from build123d import *

# Parameters (mm, degrees)
SKETCH1_R           = 150
SKETCH1_R_2         = 1.25
SKETCH1_R_3         = 1
SKETCH1_W           = 2
SKETCH1_H           = 4
BOSS_EXTRUDE1_DEPTH = 3.175
SKETCH2_R           = 1.4224
CUT_EXTRUDE1_DEPTH  = 10


with BuildPart() as part:
    # Sketch1 → Boss-Extrude1 (new body)
    with BuildSketch(Plane(origin=(0, 0, 0), x_dir=(1, 0, 0), z_dir=(0, 1, 0))):
        with Locations((106.066017178, 106.066017178)):
            Circle(SKETCH1_R)
        with Locations((77.066017178, 172.293864025)):
            Circle(SKETCH1_R_2, mode=Mode.SUBTRACT)
        with Locations((135.066017178, 172.293864025)):
            Circle(SKETCH1_R_2, mode=Mode.SUBTRACT)
        with Locations((77.066017178, 123.293864025)):
            Circle(SKETCH1_R_2, mode=Mode.SUBTRACT)
        with Locations((135.066017178, 123.293864025)):
            Circle(SKETCH1_R_2, mode=Mode.SUBTRACT)
        with Locations((95.566017178, 112.316017178)):
            Circle(SKETCH1_R_3, mode=Mode.SUBTRACT)
        with Locations((116.566017178, 112.316017178)):
            Circle(SKETCH1_R_3, mode=Mode.SUBTRACT)
        with Locations((116.566017178, 99.816017178)):
            Circle(SKETCH1_R_3, mode=Mode.SUBTRACT)
        with Locations((95.566017178, 99.816017178)):
            Circle(SKETCH1_R_3, mode=Mode.SUBTRACT)
        with Locations((172.245046965, 123.293864025)):
            Circle(SKETCH1_R_2, mode=Mode.SUBTRACT)
        with Locations((172.245046965, 179.173864025)):
            Circle(SKETCH1_R_2, mode=Mode.SUBTRACT)
        with Locations((191.295046965, 123.293864025)):
            Circle(SKETCH1_R_2, mode=Mode.SUBTRACT)
        with Locations((191.295046965, 179.173864025)):
            Circle(SKETCH1_R_2, mode=Mode.SUBTRACT)
        with Locations((98.098528615, 85.439926251)):
            Rectangle(SKETCH1_W, SKETCH1_H, mode=Mode.SUBTRACT)
        with Locations((26.098528615, 85.439926251)):
            Rectangle(SKETCH1_W, SKETCH1_H, mode=Mode.SUBTRACT)
        with Locations((98.098528615, 70.439926251)):
            Rectangle(SKETCH1_W, SKETCH1_H, mode=Mode.SUBTRACT)
        with Locations((98.098528615, 55.439926251)):
            Rectangle(SKETCH1_W, SKETCH1_H, mode=Mode.SUBTRACT)
        with Locations((98.098528615, 40.439926251)):
            Rectangle(SKETCH1_W, SKETCH1_H, mode=Mode.SUBTRACT)
        with Locations((26.098528615, 70.439926251)):
            Rectangle(SKETCH1_W, SKETCH1_H, mode=Mode.SUBTRACT)
        with Locations((26.098528615, 55.439926251)):
            Rectangle(SKETCH1_W, SKETCH1_H, mode=Mode.SUBTRACT)
        with Locations((26.098528615, 40.439926251)):
            Rectangle(SKETCH1_W, SKETCH1_H, mode=Mode.SUBTRACT)
        with Locations((114.033505741, 85.439926251)):
            Rectangle(SKETCH1_W, SKETCH1_H, mode=Mode.SUBTRACT)
        with Locations((114.033505741, 70.439926251)):
            Rectangle(SKETCH1_W, SKETCH1_H, mode=Mode.SUBTRACT)
        with Locations((114.033505741, 55.439926251)):
            Rectangle(SKETCH1_W, SKETCH1_H, mode=Mode.SUBTRACT)
        with Locations((114.033505741, 40.439926251)):
            Rectangle(SKETCH1_W, SKETCH1_H, mode=Mode.SUBTRACT)
        with Locations((186.033505741, 40.439926251)):
            Rectangle(SKETCH1_W, SKETCH1_H, mode=Mode.SUBTRACT)
        with Locations((186.033505741, 55.439926251)):
            Rectangle(SKETCH1_W, SKETCH1_H, mode=Mode.SUBTRACT)
        with Locations((186.033505741, 70.439926251)):
            Rectangle(SKETCH1_W, SKETCH1_H, mode=Mode.SUBTRACT)
        with Locations((186.033505741, 85.439926251)):
            Rectangle(SKETCH1_W, SKETCH1_H, mode=Mode.SUBTRACT)
    extrude(amount=BOSS_EXTRUDE1_DEPTH)

    # Sketch2 → Cut-Extrude1 (cut)
    with BuildSketch(Plane(origin=(0, 3.175, 0), x_dir=(1, 0, 0), z_dir=(0, 1, 0))):
        with Locations((5.303300859, 206.828733497)):
            Circle(SKETCH2_R)
        with Locations((12.374368671, 199.757665685)):
            Circle(SKETCH2_R)
        with Locations((206.828733497, 206.828733497)):
            Circle(SKETCH2_R)
        with Locations((199.757665685, 199.757665685)):
            Circle(SKETCH2_R)
        with Locations((206.828733497, 5.303300859)):
            Circle(SKETCH2_R)
        with Locations((199.757665685, 12.374368671)):
            Circle(SKETCH2_R)
        with Locations((5.303300859, 5.303300859)):
            Circle(SKETCH2_R)
        with Locations((12.374368671, 12.374368671)):
            Circle(SKETCH2_R)
        Polygon((15.432605499, 192.209300796), (13.311285156, 194.33062114), (17.801413216, 198.8207492), (19.92273356, 196.699428857), align=None)
        Polygon((-0.123743687, 207.765649982), (-2.24506403, 209.886970326), (2.24506403, 214.377098386), (4.366384374, 212.255778043), align=None)
        Polygon((192.209300796, 196.699428857), (194.33062114, 198.8207492), (198.8207492, 194.33062114), (196.699428857, 192.209300796), align=None)
        Polygon((207.765649982, 212.255778043), (209.886970326, 214.377098386), (214.377098386, 209.886970326), (212.255778043, 207.765649982), align=None)
        Polygon((196.699428857, 19.92273356), (198.8207492, 17.801413216), (194.33062114, 13.311285156), (192.209300796, 15.432605499), align=None)
        Polygon((212.255778043, 4.366384374), (214.377098386, 2.24506403), (209.886970326, -2.24506403), (207.765649982, -0.123743687), align=None)
        Polygon((19.92273356, 15.432605499), (17.801413216, 13.311285156), (13.311285156, 17.801413216), (15.432605499, 19.92273356), align=None)
        Polygon((4.366384374, -0.123743687), (2.24506403, -2.24506403), (-2.24506403, 2.24506403), (-0.123743687, 4.366384374), align=None)
    extrude(amount=-CUT_EXTRUDE1_DEPTH, mode=Mode.SUBTRACT)


solid = part.part
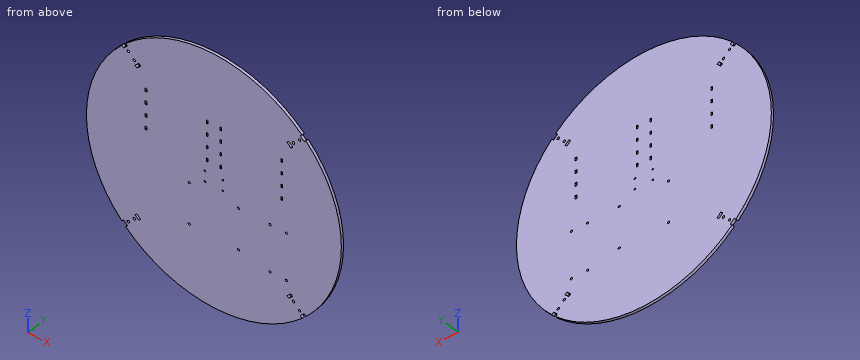
Can you work these out from the model? Positions are in its coordinate system, mm. Give positions to 0.01 mm unless a question says otherwise; leave off trailing zeros. Loops run counter-clockwise (first coordinate to the right, second up) from the corner with the lowest first, then second, coordinate; pieces in that order, holes last. Notation, with made-up numbers: M 25,60.5 L 80,60.5 A15 ccw 80,82.5 Z; hole C 36,-40 d10. An arc over 180 degrees is marked long. One line per item, written item: value. Start each with the question number.
1) If we section it at A-A, the plane y = 1.6: Give the number of separate pieces and of enclosed holes in the cut face, and give its area (3 significant figures).
2) If we section it at C-C, the plane z = -150.5: Write out the boundary of the cut face in (x, y) (3 decimals).
3) I'm going to push flat-ended pins straight in: pin 1 (1.5 mm diameter, centred on x = 172.25, z = -179.17, fed in from -Y); pin 2 (1 mm diameter, centred on x = 186, y = 1.5, fed in from -Z); pin 3 (1.6 mm diameter, centred on y = 1.5, z = -55, fed in from -X). Where does each tip first touch, or does it pass through?
4) If we section it at B-B, the plane x = 31.5: Write out the boundary of the cut face in (y, z) (3 decimals).
5) If I drill on line 1 (Z direction, x = 97.5, y = 1.9); line 2 (Z direction, x = 218.5, y = 1.45); line 3 (Z direction, x = 15, y = 1), over which ranges is the centre line in solid material (lowest first)? Write a range as [from, to].
Completed:
1. separate pieces: 1
1. enclosed holes: 40
1. area: 70,300 mm^2
2. outline: M -37.202,0 L 249.334,0 L 249.334,3.175 L -37.202,3.175 Z
3. pin 1: passes through
3. pin 2: stops at z = -233.31
3. pin 3: stops at x = -35.26
4. outline: M 0,-236.219 L 3.175,-236.219 L 3.175,24.087 L 0,24.087 Z
5. line 1: z = [-255.82, -87.44], [-83.44, -72.44], [-68.44, -57.44], [-53.44, -42.44], [-38.44, 43.69]
5. line 2: z = [-205.36, -6.78]
5. line 3: z = [-225.26, -196.02], [-192.64, -19.49], [-16.11, 13.13]
